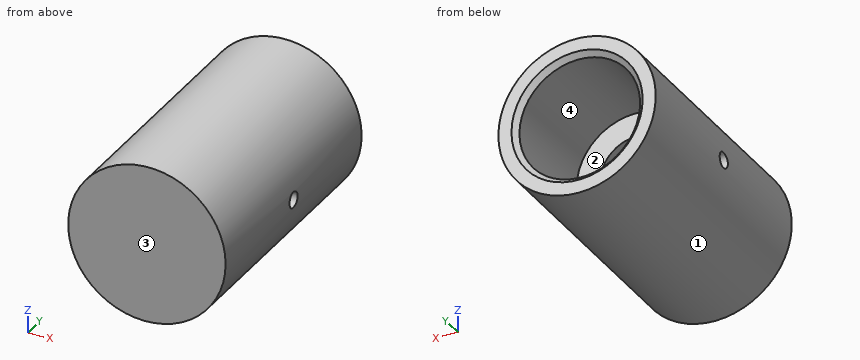
```python
from build123d import *

# Parameters (mm, degrees)
SKETCH1_R                      = 7.5
BOSS_EXTRUDE1_DEPTH            = 25
SKETCH2_R                      = 5.75
CUT_EXTRUDE1_DEPTH             = 11
CHAMFER1_SIZE                  = 0.5
SKETCH3_R                      = 3.5
CUT_EXTRUDE2_DEPTH             = 10
CUT_EXTRUDE3_REACH             = 9.5
SKETCH4_R                      = 0.75
CUT_EXTRUDE3_DIRECTION_2_REACH = 9.5


with BuildPart() as part:
    # Sketch1 → Boss-Extrude1 (new body)
    with BuildSketch(Plane(origin=(0, 0, 0), x_dir=(1, 0, 0), z_dir=(0, 1, 0))):
        Circle(SKETCH1_R)
    extrude(amount=BOSS_EXTRUDE1_DEPTH)

    # Sketch2 → Cut-Extrude1 (cut)
    with BuildSketch(Plane(origin=(0, 25, 0), x_dir=(1, 0, 0), z_dir=(0, 1, 0))):
        Circle(SKETCH2_R)
    extrude(amount=-CUT_EXTRUDE1_DEPTH, mode=Mode.SUBTRACT)

    # Chamfer1
    chamfer1_edges = [part.edges().sort_by_distance(p)[0] for p in [
        (-5.75, 25, 0),
    ]]
    chamfer(chamfer1_edges, length=CHAMFER1_SIZE)

    # Sketch3 → Cut-Extrude2 (cut)
    with BuildSketch(Plane(origin=(0, 14, 0), x_dir=(1, 0, 0), z_dir=(0, 1, 0))):
        Circle(SKETCH3_R)
    extrude(amount=-CUT_EXTRUDE2_DEPTH, mode=Mode.SUBTRACT)

    # Sketch4 → Cut-Extrude3 (cut, up to next)
    with BuildSketch(Plane(origin=(0, 0, 0), x_dir=(0, 0, -1), z_dir=(1, 0, 0)), mode=Mode.PRIVATE) as cut_extrude3_sk1:
        with Locations((0, 12.5)):
            Circle(SKETCH4_R)
    cut_extrude3_tool1 = extrude(cut_extrude3_sk1.sketch, amount=-CUT_EXTRUDE3_REACH, mode=Mode.PRIVATE) & part.part
    add(cut_extrude3_tool1.solids().sort_by_distance((0, 12.5, 0))[0], mode=Mode.SUBTRACT)

    # Sketch4 → Cut-Extrude3 direction 2 (cut, up to next)
    with BuildSketch(Plane(origin=(0, 0, 0), x_dir=(0, 0, -1), z_dir=(1, 0, 0)), mode=Mode.PRIVATE) as cut_extrude3_direction_2_sk1:
        with Locations((0, 12.5)):
            Circle(SKETCH4_R)
    cut_extrude3_direction_2_tool1 = extrude(cut_extrude3_direction_2_sk1.sketch, amount=CUT_EXTRUDE3_DIRECTION_2_REACH, mode=Mode.PRIVATE) & part.part
    add(cut_extrude3_direction_2_tool1.solids().sort_by_distance((0, 12.5, 0))[0], mode=Mode.SUBTRACT)


solid = part.part
```
Geometry check sheet. Reference: the model listing, model coordinates, mm. Face numbers are marked on the shaded views. Coordinates: 2 decimals unless noted, no trailing zeros. Write each loop counter-clockwise with the first axis right and the second up, starting at its lowest first coordinate (ties: lowest second). Pieces come first, ordered by that corner, then holes. Notation, with made-up numbers: M 52.5,-23.5 L 100.5,-23.5 A20 cw 100.5,-10.5 Z; hole C 69,21.25 d7. An arc over 180 degrees is marked long. Use one line per item in the form item = value. Start each with the question number.
1) Go/stop test with flat-tipped pins: pin 1 Ø5.5 at (x, z) = (0, 0) entering from +Y; pin 2 Ø6 at (x, z) = (-6, 4) entering from -Y; pin 3 Ø3 at (y, z) = (16, 2) entering from -X; pin 4 Ø3 at (x, y) = (3, 3) entering from +Z. Record where each tip stops, or that it passes through.
2) Thickness scan on probe 1 along Z at (x, y) = (0, 7); probe 2 along Y at (x, z) = (-5.45, 0); probe 3 along Y at (x, z) = (-6.6, 0). Record the ranges inside material, lowest first. Write a range as from..to.
3) Section check B-B on x = 0. Enter the section's corners in (y, z), and give its area (3 significant figures).
4) Release check for a two-part mould opening along Z. For the marked faces 1, 2, 3 and 4 record: pulls with the +Z half, pulls with the -Z half, needs draft (parallel to the pull), parting line crosses it, or undercut.
5) Section check A-A on z = 0. Enter the section's corners in (x, y), and give its area (3 significant figures).
6) Section check C-C on y = 12.5. Enter the section's corners in (x, z), and give its area (3 significant figures).
7) Section check D-D on y = 20.25. Enter the section's corners in (x, z), and give its area (3 significant figures).
Responses:
q1.pin_1 = 4
q1.pin_2 = 0
q1.pin_3 = -7.48
q1.pin_4 = 7.35
q2.probe_1 = -7.5..-3.5, 3.5..7.5
q2.probe_2 = 0..11.75, 13.25..14
q2.probe_3 = 0..11.75, 13.25..25
q3.outline = M 0,-7.5 L 25,-7.5 L 25,-6.25 L 24.5,-5.75 L 14,-5.75 L 14,-3.5 L 4,-3.5 L 4,3.5 L 14,3.5 L 14,5.75 L 24.5,5.75 L 25,6.25 L 25,7.5 L 0,7.5 Z
q3.area = 178 mm2
q4.face_1 = parting line crosses it
q4.face_2 = undercut
q4.face_3 = needs draft
q4.face_4 = undercut
q5.outline = M -7.5,0 L 7.5,0 L 7.5,11.75 L 3.5,11.75 L 3.5,4 L -3.5,4 L -3.5,11.75 L -7.5,11.75 Z; M -7.5,13.25 L -3.5,13.25 L -3.5,14 L -5.75,14 L -5.75,24.5 L -6.25,25 L -7.5,25 Z; M 3.5,13.25 L 7.5,13.25 L 7.5,25 L 6.25,25 L 5.75,24.5 L 5.75,14 L 3.5,14 Z
q5.area = 166 mm2
q6.outline = M -7.46,-0.75 A7.5 ccw 7.46,-0.75 L 3.42,-0.75 A3.5 cw -3.42,-0.75 Z; M -7.46,0.75 L -3.42,0.75 A3.5 cw 3.42,0.75 L 7.46,0.75 A7.5 ccw Z
q6.area = 126 mm2
q7.outline = C 0,0 d15; hole C 0,0 d11.5
q7.area = 72.8 mm2
